Model file for the job. Use its own axes, mm. A direction names the side the tool comes from. Give positions to 0.01 mm unless a question says otherwise; leave off trailing zeros. Loops run counter-clockwise (first coordinate to the right, second up) from the corner with the lowest first, then second, coordinate; pieces in that order, holes last. Notation, with made-up numbers: (-6, 37) - (35, 37) arc R16 ccw to (35, 58) - close; hole circle Ø11 at (6.5, -33). An arc over 180 degrees is marked (long way). Answer as CSV lines item,"result". Start each with the question number.
Item 1: Saw through at A-A on z = 236. Give the cut face in (x, y).
Item 2: Pull direction Y, two halves, no side cores. Call faces 3 (the flat face through (-3, 3, 0)), 4 (the flat face through (-107, 1, 6)), 5 (the flat face through (-3, 230, 138)): pulls with the +Y half, pulls with the -Y half, needs draft (parallel to the pull), parting line crosses it, or undercut.
Item 3: Tool access for faces 1 (the flat face through (-107, -78.667, 105)), 2 (the flat face through (215, -3, 138)): list every direction of +Z, -Z, +X, -X, +Y, -Y with a clear straight run to the whole face (end or side of a thin tool).
Item 4: Pin check, flat tip, straight feed: pin 1 (10 mm diameter, centred on x = -70, y = -153.5, fed in from +Z). Stop position of the tip, or through.
Item 5: Drill centre lines: L1, parallel to X at y = 85.5, z = 205.5; L2, parallel to Y at x = -14, z = 24; L3, parallel to X at y = -110, z = 246. Where is each one in solid material? Low to high. Write a range as from..to.
Item 6: Saw through at B-B on x = 18. Give the cut face in (y, z).
Item 7: Saw through at D-D on z = 195.5. Give the cut face in (x, y), plus the area to 3 significant figures.
Item 8: Saw through at C-C on y = -164. Give the cut face in (x, z), plus the area to 3 significant figures.
from build123d import *

# Parameters (mm, degrees)
F0_W     = 430
F0_H     = 460
F1_DEPTH = 280
F2_T     = -6
F4_DEPTH = 460.001
F5_W     = 206
F5_H     = 6
F6_DEPTH = 200


with BuildPart() as f1:
    # F0 (on Top) → F1 (new body)
    with BuildSketch(Plane.XY):
        Rectangle(F0_W, F0_H)
    extrude(amount=F1_DEPTH)

    # F2
    f2_openings = [f1.faces().sort_by_distance(p)[0] for p in [
        (0, 0, 280),
    ]]
    offset(amount=F2_T, openings=f2_openings)

    # F3 (on face) → F4 (cut, through all)
    with BuildSketch(Plane.XZ.offset(230)):
        with BuildLine():
            ThreePointArc((31.061347, 222.770627), (49.67535, 235.90859), (37.579824, 255.216242))
            ThreePointArc((37.579824, 255.216242), (0, 260), (-37.579824, 255.216242))
            ThreePointArc((-37.579824, 255.216242), (-49.67535, 235.90859), (-31.061347, 222.770627))
            ThreePointArc((-31.061347, 222.770627), (0, 225), (31.061347, 222.770627))
        make_face()
    extrude(amount=-F4_DEPTH, mode=Mode.SUBTRACT)

    # F5 (on face) → F6 (join)
    with BuildSketch(Plane.XY.offset(6)):
        Polygon((3, 78.666667), (3, 224), (-3, 224), (-3, 78.666667), (-3, 72.666667), (-3, -72.666667), (-3, -78.666667), (-3, -224), (3, -224), (3, -78.666667), (3, -72.666667), (3, 72.666667), align=None)
        with Locations((106, 75.666667)):
            Rectangle(F5_W, F5_H)
        with Locations((-106, 75.666667)):
            Rectangle(F5_W, F5_H)
        with Locations((106, -75.666667)):
            Rectangle(F5_W, F5_H)
        with Locations((-106, -75.666667)):
            Rectangle(F5_W, F5_H)
    extrude(amount=F6_DEPTH)


solid = f1.part
Responses:
1,outline,"(-215, -230) - (-49.69, -230) - (-49.69, -224) - (-209, -224) - (-209, 224) - (-49.69, 224) - (-49.69, 230) - (-215, 230) - close; (49.69, -230) - (215, -230) - (215, 230) - (49.69, 230) - (49.69, 224) - (209, 224) - (209, -224) - (49.69, -224) - close"
2,face 3,"needs draft"
2,face 4,"undercut"
2,face 5,"pulls with the +Y half"
3,face 1,"+Z"
3,face 2,"+Z, -Z, +X, +Y, -Y"
4,pin 1,"z = 6"
5,L1,"-215..-209, -3..3, 209..215"
5,L2,"-230..-224, -78.67..-72.67, 72.67..78.67, 224..230"
5,L3,"-215..-209, 209..215"
6,outline,"(-230, 0) - (230, 0) - (230, 224.25) - (224, 224.25) - (224, 6) - (78.67, 6) - (78.67, 206) - (72.67, 206) - (72.67, 6) - (-72.67, 6) - (-72.67, 206) - (-78.67, 206) - (-78.67, 6) - (-224, 6) - (-224, 224.25) - (-230, 224.25) - close; (-230, 258.92) - (-224, 258.92) - (-224, 280) - (-230, 280) - close; (224, 258.92) - (230, 258.92) - (230, 280) - (224, 280) - close"
7,outline,"(-215, -230) - (215, -230) - (215, 230) - (-215, 230) - close; hole (-209, -224) - (-3, -224) - (-3, -78.67) - (-209, -78.67) - close; hole (-209, -72.67) - (-3, -72.67) - (-3, 72.67) - (-209, 72.67) - close; hole (-209, 78.67) - (-3, 78.67) - (-3, 224) - (-209, 224) - close; hole (3, -224) - (209, -224) - (209, -78.67) - (3, -78.67) - close; hole (3, -72.67) - (209, -72.67) - (209, 72.67) - (3, 72.67) - close; hole (3, 78.67) - (209, 78.67) - (209, 224) - (3, 224) - close"
7,area,"18,200 mm2"
8,outline,"(-215, 0) - (215, 0) - (215, 280) - (209, 280) - (209, 6) - (3, 6) - (3, 206) - (-3, 206) - (-3, 6) - (-209, 6) - (-209, 280) - (-215, 280) - close"
8,area,"7,070 mm2"
